Work out the finished part from the listing and answer in its coordinate system (mm). A direction names the side the tool comes from. Give positions to 0.01 mm unless a question says otherwise; leave off trailing zeros. Order: outer loops, then holes, each group sorted by start corner. A loop starts at its lowest first (then second) coordinate and runs counter-clockwise, first axis right, second up.
```python
from build123d import *

# Parameters (mm, degrees)
F1_DEPTH      = 9
F1_DEPTH_BACK = 5
F2_R          = 4
F3_DEPTH      = 1.27
F5_DEPTH      = 25.2476


with BuildPart() as f1:
    # F0 (on Front) → F1 (new body, two sides)
    with BuildSketch(Plane.XZ) as f1_sk:
        with BuildLine():
            ThreePointArc((4.518019, -1.1), (4.616887, -0.553945), (4.65, 0))
            ThreePointArc((4.65, 0), (4.616887, 0.553945), (4.518019, 1.1))
            ThreePointArc((4.518019, 1.1), (4.422413, 1.436929), (4.301718, 1.765707))
            ThreePointArc((4.301718, 1.765707), (3.761929, 2.733201), (3.008591, 3.545544))
            ThreePointArc((3.008591, 3.545544), (2.733201, 3.761929), (2.442307, 3.956973))
            ThreePointArc((2.442307, 3.956973), (1.436929, 4.422413), (0.349983, 4.636811))
            ThreePointArc((0.349983, 4.636811), (0, 4.65), (-0.349983, 4.636811))
            ThreePointArc((-0.349983, 4.636811), (-1.436929, 4.422413), (-2.442307, 3.956973))
            ThreePointArc((-2.442307, 3.956973), (-2.733201, 3.761929), (-3.008591, 3.545544))
            ThreePointArc((-3.008591, 3.545544), (-3.761929, 2.733201), (-4.301718, 1.765707))
            ThreePointArc((-4.301718, 1.765707), (-4.422413, 1.436929), (-4.518019, 1.1))
            ThreePointArc((-4.518019, 1.1), (-4.65, 0), (-4.518019, -1.1))
            ThreePointArc((-4.518019, -1.1), (-4.422413, -1.436929), (-4.301718, -1.765707))
            ThreePointArc((-4.301718, -1.765707), (-3.761929, -2.733201), (-3.008591, -3.545544))
            ThreePointArc((-3.008591, -3.545544), (-2.733201, -3.761929), (-2.442307, -3.956973))
            ThreePointArc((-2.442307, -3.956973), (-1.436929, -4.422413), (-0.349983, -4.636811))
            ThreePointArc((-0.349983, -4.636811), (0, -4.65), (0.349983, -4.636811))
            ThreePointArc((0.349983, -4.636811), (1.436929, -4.422413), (2.442307, -3.956973))
            ThreePointArc((2.442307, -3.956973), (2.733201, -3.761929), (3.008591, -3.545544))
            ThreePointArc((3.008591, -3.545544), (3.761929, -2.733201), (4.301718, -1.765707))
            ThreePointArc((4.301718, -1.765707), (4.422413, -1.436929), (4.518019, -1.1))
        make_face()
        with BuildLine():
            ThreePointArc((4.518019, 1.1), (4.616887, 0.553945), (4.65, 0))
            ThreePointArc((4.65, 0), (4.616887, -0.553945), (4.518019, -1.1))
            Line((4.518019, -1.1), (4.618019, -1.1))
            Line((4.618019, -1.1), (6.25, -0.329923))
            Line((6.25, -0.329923), (6.25, 0))
            Line((6.25, 0), (6.25, 0.329923))
            Line((6.25, 0.329923), (4.618019, 1.1))
            Line((4.618019, 1.1), (4.518019, 1.1))
        make_face()
        with BuildLine():
            ThreePointArc((3.008591, 3.545544), (3.761929, 2.733201), (4.301718, 1.765707))
            Line((4.301718, 1.765707), (4.38262, 1.824485))
            Line((4.38262, 1.824485), (5.25028, 3.406744))
            Line((5.25028, 3.406744), (5.056356, 3.673658))
            Line((5.056356, 3.673658), (4.862432, 3.940572))
            Line((4.862432, 3.940572), (3.089492, 3.604322))
            Line((3.089492, 3.604322), (3.008591, 3.545544))
        make_face()
        with BuildLine():
            Line((4.38262, -1.824485), (4.301718, -1.765707))
            ThreePointArc((4.301718, -1.765707), (3.761929, -2.733201), (3.008591, -3.545544))
            Line((3.008591, -3.545544), (3.089492, -3.604322))
            Line((3.089492, -3.604322), (4.862432, -3.940572))
            Line((4.862432, -3.940572), (5.056356, -3.673658))
            Line((5.056356, -3.673658), (5.25028, -3.406744))
            Line((5.25028, -3.406744), (4.38262, -1.824485))
        make_face()
        with BuildLine():
            ThreePointArc((0.349983, 4.636811), (1.436929, 4.422413), (2.442307, 3.956973))
            Line((2.442307, 3.956973), (2.473209, 4.052079))
            Line((2.473209, 4.052079), (2.245132, 5.842151))
            Line((2.245132, 5.842151), (1.931356, 5.944103))
            Line((1.931356, 5.944103), (1.61758, 6.046055))
            Line((1.61758, 6.046055), (0.380884, 4.731916))
            Line((0.380884, 4.731916), (0.349983, 4.636811))
        make_face()
        with BuildLine():
            Line((2.473209, -4.052079), (2.442307, -3.956973))
            ThreePointArc((2.442307, -3.956973), (1.436929, -4.422413), (0.349983, -4.636811))
            Line((0.349983, -4.636811), (0.380884, -4.731916))
            Line((0.380884, -4.731916), (1.61758, -6.046055))
            Line((1.61758, -6.046055), (1.931356, -5.944103))
            Line((1.931356, -5.944103), (2.245132, -5.842151))
            Line((2.245132, -5.842151), (2.473209, -4.052079))
        make_face()
        with BuildLine():
            ThreePointArc((-2.442307, 3.956973), (-1.436929, 4.422413), (-0.349983, 4.636811))
            Line((-0.349983, 4.636811), (-0.380884, 4.731916))
            Line((-0.380884, 4.731916), (-1.61758, 6.046055))
            Line((-1.61758, 6.046055), (-1.931356, 5.944103))
            Line((-1.931356, 5.944103), (-2.245132, 5.842151))
            Line((-2.245132, 5.842151), (-2.473209, 4.052079))
            Line((-2.473209, 4.052079), (-2.442307, 3.956973))
        make_face()
        with BuildLine():
            Line((-0.380884, -4.731916), (-0.349983, -4.636811))
            ThreePointArc((-0.349983, -4.636811), (-1.436929, -4.422413), (-2.442307, -3.956973))
            Line((-2.442307, -3.956973), (-2.473209, -4.052079))
            Line((-2.473209, -4.052079), (-2.245132, -5.842151))
            Line((-2.245132, -5.842151), (-1.931356, -5.944103))
            Line((-1.931356, -5.944103), (-1.61758, -6.046055))
            Line((-1.61758, -6.046055), (-0.380884, -4.731916))
        make_face()
        with BuildLine():
            ThreePointArc((-4.301718, 1.765707), (-3.761929, 2.733201), (-3.008591, 3.545544))
            Line((-3.008591, 3.545544), (-3.089492, 3.604322))
            Line((-3.089492, 3.604322), (-4.862432, 3.940572))
            Line((-4.862432, 3.940572), (-5.056356, 3.673658))
            Line((-5.056356, 3.673658), (-5.25028, 3.406744))
            Line((-5.25028, 3.406744), (-4.38262, 1.824485))
            Line((-4.38262, 1.824485), (-4.301718, 1.765707))
        make_face()
        with BuildLine():
            Line((-3.089492, -3.604322), (-3.008591, -3.545544))
            ThreePointArc((-3.008591, -3.545544), (-3.761929, -2.733201), (-4.301718, -1.765707))
            Line((-4.301718, -1.765707), (-4.38262, -1.824485))
            Line((-4.38262, -1.824485), (-5.25028, -3.406744))
            Line((-5.25028, -3.406744), (-5.056356, -3.673658))
            Line((-5.056356, -3.673658), (-4.862432, -3.940572))
            Line((-4.862432, -3.940572), (-3.089492, -3.604322))
        make_face()
        with BuildLine():
            ThreePointArc((-4.518019, -1.1), (-4.65, 0), (-4.518019, 1.1))
            Line((-4.518019, 1.1), (-4.618019, 1.1))
            Line((-4.618019, 1.1), (-6.25, 0.329923))
            Line((-6.25, 0.329923), (-6.25, 0))
            Line((-6.25, 0), (-6.25, -0.329923))
            Line((-6.25, -0.329923), (-4.618019, -1.1))
            Line((-4.618019, -1.1), (-4.518019, -1.1))
        make_face()
    extrude(amount=F1_DEPTH)
    extrude(f1_sk.sketch, amount=-F1_DEPTH_BACK)

    # F2 (on face) → F3 (join)
    with BuildSketch(Plane.XZ.offset(9)):
        Circle(F2_R)
    extrude(amount=F3_DEPTH)

    # F4 (on face) → F5 (cut)
    with BuildSketch(Plane.XZ.offset(10.27)):
        with BuildLine():
            Line((1.322876, 1.5), (-1.322876, 1.5))
            ThreePointArc((-1.322876, 1.5), (0, -2), (1.322876, 1.5))
        make_face()
    extrude(amount=-F5_DEPTH, mode=Mode.SUBTRACT)


solid = f1.part
```
1. The part is cut by section B-B (z = 0). Write down the section's boundary in (x, y).
Findings below:
outline: (-6.25, -9) - (-4, -9) - (-4, -10.27) - (-2, -10.27) - (-2, 5) - (-6.25, 5) - close; (2, -10.27) - (4, -10.27) - (4, -9) - (6.25, -9) - (6.25, 5) - (2, 5) - close
2. The mould has two halves that part along Z. Classify faces 1 (the face through (-2.358, -2.098, 4.96)), 2 (the face through (-5.42, -2.1, 0.72)), 3 (the face through (-0.867, -9.626, -3.905)), 4 (the face through (0, -10.27, 2)): pulls with the +Z half, pulls with the -Z half, needs draft (parallel to the pull), parting line crosses it, or undercut.
Findings below:
face 1: pulls with the +Z half
face 2: undercut
face 3: parting line crosses it
face 4: needs draft
3. Which of the six approach directions +Z, -Z, +X, -X, +Y, -Y give full straight-line access (tool end or side, diameter ignored) to faces 5 (the face through (1.01, -2.1, 5.4)), 6 (the face through (0, -3, 1.5)), 7 (the face through (-4.81, -2.1, -2.6)), 8 (the face through (5.445, -2.098, 0.71))?
Findings below:
face 5: +Z, +Y, -Y
face 6: +Y, -Y
face 7: -X, +Y, -Y
face 8: +X, +Y, -Y
4. Straight lines are drawn through the part: probe 1 along X at (y, z) = (2.25, 0); probe 2 along Z at (x, y) = (-5, -8.5); probe 3 along Z at (x, y) = (4.75, 3.5). For each, find the intervals that lie inside material, in ascending order.
Findings below:
probe 1: x = -6.25 to -2, 2 to 6.25
probe 2: z = -3.75 to -2.95, -0.92 to 0.92, 2.95 to 3.75
probe 3: z = -3.92 to -2.49, -1.04 to 1.04, 2.49 to 3.92
5. Given P1, Ø1, axis at y = 3, z = 2.5, coming from the -X side; P2, Ø3, axis at x = 3.5, y = -6, coming from the -Z side; P3, Ø6, axis at y = -7, z = 4, coming from the +X side, each flat-ended and moving along its own axis, determine where each tip first touches the part or whether it passes through.
Findings below:
P1: stops at x = -5.03
P2: stops at z = -5.92
P3: stops at x = 5.25
6. The part is cut by section A-A (x = 0). Write down the section's boundary in (y, z).
Findings below:
outline: (-10.27, -4) - (-9, -4) - (-9, -4.65) - (5, -4.65) - (5, -2) - (-10.27, -2) - close; (-10.27, 1.5) - (5, 1.5) - (5, 4.65) - (-9, 4.65) - (-9, 4) - (-10.27, 4) - close
